Input: dimensioned drawing with shaded views. Units: mm. Origin: part minimum x, y, z. A direction names the side the tool comes from. Round coordinates to 2 decimals unless told otherwise and drop trailing zeros. Order: outer loops, then holes, each group sorted by start corner. A loop starts at its lowest first (then second) coordinate and runs counter-clockwise, first axis right, second up. Notation, with made-up numbers: (61, 64) - (86, 64) arc R22 cw to (86, 71) - close; hole circle Ø3 at (-9.5, 33.5). An arc over 180 degrees is marked (long way). One line per item, written item: value. Start each with the question number.
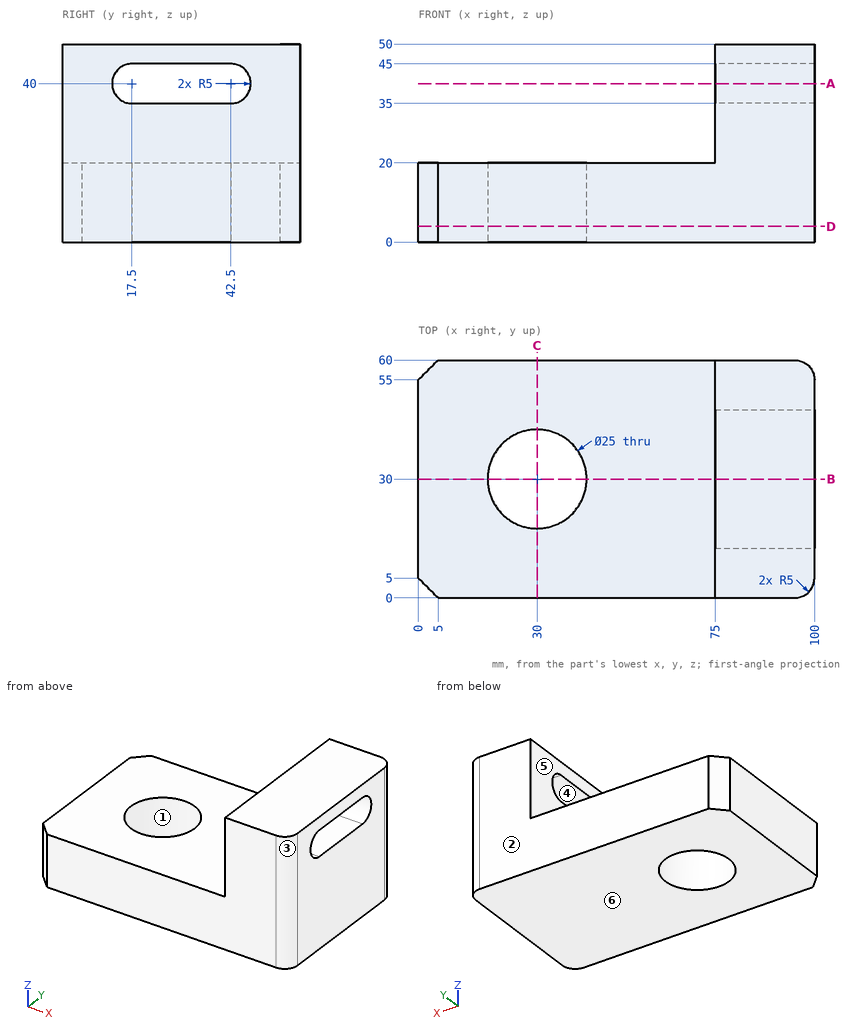
1. Set-up query: the marked faces 4, 5 and 6. Return all of +Z, -Z, +X, -X, +Y, -Y with unobstructed straight access to the full face (end or side cutting, diameter ignored); none if empty.
2. Pin query (flat end, axial travel): pin 1 (20 mm diameter, centred on x = 30, y = 30, fed in from +Z); pin 2 (2 mm diameter, centred on y = 36.5, z = 27.5, fed in from -X); pin 3 (24 mm diameter, centred on y = 26.5, z = 28.5, fed in from -X); pin 4 (18 mm diameter, centred on x = 40, y = 43.5, fed in from +Z). Return the tip coordinate at first contact, or that it passes through.
3. Section B-B (y = 30). Return the cut outline in (x, z), then the cut area to 3 significant figures.
4. Line query: line 1 (Y direction, x = 30, z = 12); line 2 (Z direction, x = 81, y = 37); line 3 (Z direction, x = 41, y = 53). Output: solid intervals per line, ascending. Write a range as from..to.
5. Pull-direction query (Y, two-part tool) for the marked faces 1, 2 and 3; classes: released by +Y, released by -Y, zero draft, split by the parting line, or undercut.
6. Section C-C (x = 30). Return the cut outline in (y, z), then the cut area to 3 significant figures.
7. Section A-A (z = 40). Return the cut outline in (x, y).
8. Section D-D (z = 4). Return the cut outline in (x, y).
Solved:
1. face 4: +X, -X
1. face 5: +Z, -X, +Y, -Y
1. face 6: -Z, +X, -X, +Y, -Y
2. pin 1: passes through
2. pin 2: stops at x = 75
2. pin 3: stops at x = 0
2. pin 4: stops at z = 20
3. outline: (0, 0) - (17.5, 0) - (17.5, 20) - (0, 20) - close; (42.5, 0) - (100, 0) - (100, 35) - (75, 35) - (75, 20) - (42.5, 20) - close; (75, 45) - (100, 45) - (100, 50) - (75, 50) - close
3. area: 2,000 mm²
4. line 1: y = 0..17.5, 42.5..60
4. line 2: z = 0..35, 45..50
4. line 3: z = 0..20
5. face 1: undercut
5. face 2: released by +Y
5. face 3: released by -Y
6. outline: (0, 0) - (17.5, 0) - (17.5, 20) - (0, 20) - close; (42.5, 0) - (60, 0) - (60, 20) - (42.5, 20) - close
6. area: 700 mm²
7. outline: (75, 0) - (95, 0) arc R5 ccw to (100, 5) - (100, 12.5) - (75, 12.5) - close; (75, 47.5) - (100, 47.5) - (100, 55) arc R5 ccw to (95, 60) - (75, 60) - close
8. outline: (0, 5) - (5, 0) - (95, 0) arc R5 ccw to (100, 5) - (100, 55) arc R5 ccw to (95, 60) - (5, 60) - (0, 55) - close; hole circle Ø25 at (30, 30)
